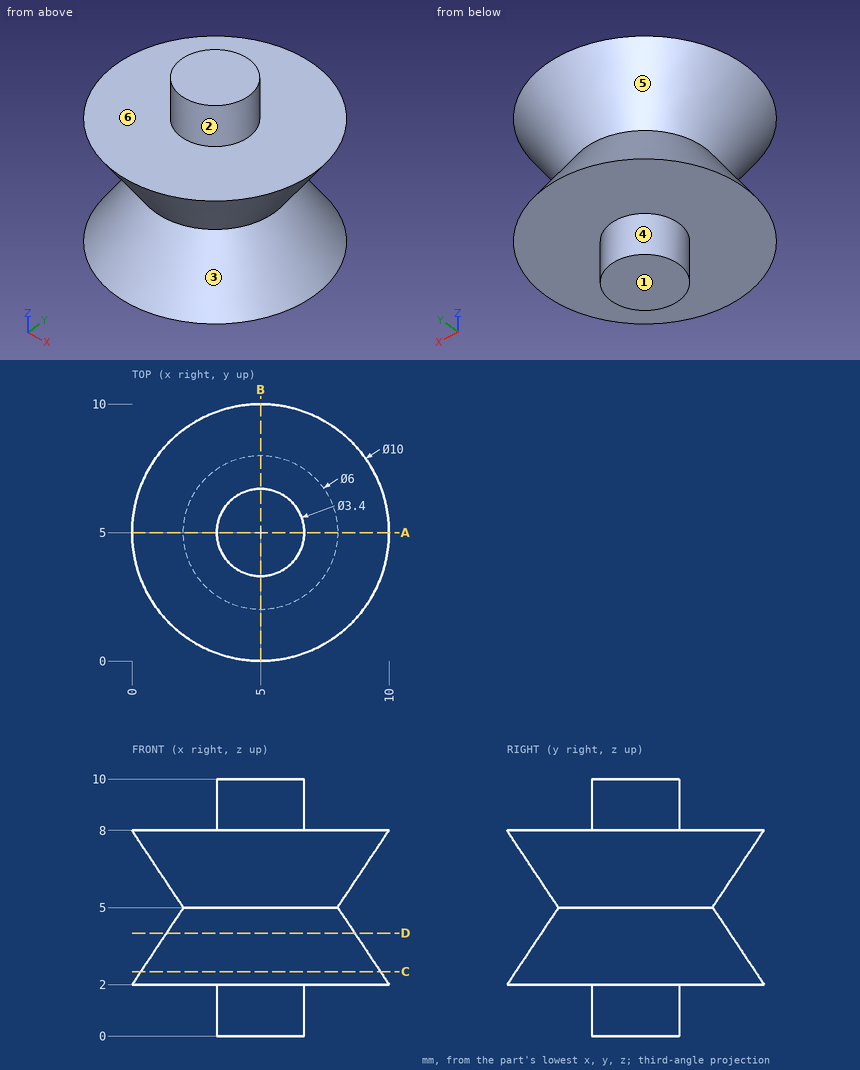
Study the drawing (mm; zero at the part's minimum x, y, z) and answer. A direction names the side the tool comes from. Round coordinates to 2 decimals unless told otherwise and drop trailing zeros. Write each loop counter-clockwise with the first axis right and the second up, starting at its lowest first coordinate (ties: lowest second). Pieces come first, ordered by that corner, then holes. Notation, with made-up numbers: (-25.5, 67) -> (26.5, 67) arc R33 ccw to (26.5, 95) -> close; hole circle Ø8 at (-5.5, -35). An arc over 180 degrees is marked (long way). Write item = value, one per line.
1) Section C-C on z = 2.5 is taken. Write down the section's boundary in (x, y), plus the area to 3 significant figures.
Check values:
outline = circle Ø9.33 at (5, 5)
area = 68.4 mm²
2) Straight lines are drawn through the part: line 1 along Z through (x, y) = (7.25, 1.25); line 2 along Z through (x, y) = (9, 4.25); line 3 along Z through (x, y) = (2.75, 4.5). For each, find the intervals that lie inside material, in ascending order. Write a range as [from, to].
Check values:
line_1 = [2, 2.94], [7.06, 8]
line_2 = [2, 3.4], [6.6, 8]
line_3 = [2, 8]
3) Given pin 1 (1 mm diameter, centred on x = 8, y = 7, fed in from +Z); pin 2 (2 mm diameter, centred on y = 1.5, z = 6, fed in from -X); pin 3 (3 mm diameter, centred on x = 5.5, z = 4, fed in from +Y), each flat-ended and moving along its own axis, determine where each tip first touches the part or whether it passes through.
Check values:
pin_1 = 8
pin_2 = 1.95
pin_3 = 9.65
4) Section D-D on z = 4 is taken. Write down the section's boundary in (x, y), plus the area to 3 significant figures.
Check values:
outline = circle Ø7.33 at (5, 5)
area = 42.2 mm²
5) For a pull along Z with two mould halves and no side action, classify the marked faces 1, 2 and 3 as released by +Z, released by -Z, zero draft, split by the parting line, or undercut.
Check values:
face_1 = released by -Z
face_2 = zero draft
face_3 = undercut
6) Section A-A on y = 5 is taken. Write down the section's boundary in (x, z).
Check values:
outline = (0, 2) -> (3.3, 2) -> (3.3, 0) -> (6.7, 0) -> (6.7, 2) -> (10, 2) -> (8, 5) -> (10, 8) -> (6.7, 8) -> (6.7, 10) -> (3.3, 10) -> (3.3, 8) -> (0, 8) -> (2, 5) -> close
7) Which of the six approach directions +Z, -Z, +X, -X, +Y, -Y give full straight-line access (tool end or side, diameter ignored) to the marked faces 4, 5 and 6?
Check values:
face_4 = -Z
face_5 = none
face_6 = +Z
